Read the model definition and answer for the solid it produces. Units are mm, in the model's axes. A direction names the side the tool comes from. Give positions to 0.01 mm unless a question says otherwise; leave off trailing zeros. Order: outer loops, then holes, each group sorted by start corner. A loop starts at its lowest first (then second) coordinate and runs counter-clockwise, first axis right, second up.
Autodesk Inventor part; units mm, degrees
ref_plane "YZ Plane" through (0, 0, 0) normal (1, 0, 0) x (0, 1, 0)
ref_plane "XZ Plane" through (0, 0, 0) normal (0, 1, 0) x (-1, 0, 0)
ref_plane "XY Plane" through (0, 0, 0) normal (0, 0, 1) x (1, 0, 0)
sketch "Sketch1" plane through (0, 0, 0) normal (0, 1, 0) x (-1, 0, 0)
  line L0 (28, 44) -> (-28, 44)
  line L1 (-30, 42) -> (-30, -42)
  line L2 (-28, -44) -> (28, -44)
  line L3 (30, -42) -> (30, 42)
  line L4 (30, 44) -> (-30, -44) construction
  line L5 (-30, 44) -> (30, -44) construction
  line L6 (25, 42.5) -> (-25, 42.5)
  line L7 (-28, 39.5) -> (-28, -39.5)
  line L8 (-25, -42.5) -> (25, -42.5)
  line L9 (28, -39.5) -> (28, 39.5)
  line L10 (28, 42.5) -> (-28, -42.5) construction
  line L11 (-28, 42.5) -> (28, -42.5) construction
  arc A0 (25, -42.5) -> (28, -39.5) centre (25, -39.5) ccw
  arc A1 (-28, -39.5) -> (-25, -42.5) centre (-25, -39.5) ccw
  arc A2 (-25, 42.5) -> (-28, 39.5) centre (-25, 39.5) ccw
  arc A3 (28, 39.5) -> (25, 42.5) centre (25, 39.5) ccw
  arc A4 (-30, -42) -> (-28, -44) centre (-28, -42) ccw
  arc A5 (-28, 44) -> (-30, 42) centre (-28, 42) ccw
  arc A6 (28, -44) -> (30, -42) centre (28, -42) ccw
  arc A7 (30, 42) -> (28, 44) centre (28, 42) ccw
  point P0 (0, 0)
  dimension "d2" = 60
  dimension "d3" = 88
  dimension "d4" = 56
  dimension "d5" = 85
  dimension "d6" = 3
  dimension "d7" = 2
extrude "Extrusion1" add sketch "Sketch1" along normal blind 4 contours A7 L3 A6 L2 A4 L1 A5 L0 | A3 L9 A0 L8 A1 L7 A2 L6
extrude "Extrusion2" add sketch "Sketch1" against normal blind 8
sketch "Sketch2" plane through (28, 4, -44) normal (0, 0, -1) x (-1, 0, 0)
  line L0 (53, -12) -> (3, -12)
  line L1 (2, -1) -> (54, -1)
  line L2 (54, -1) -> (54, -12)
  line L3 (54, -12) -> (2, -12)
  line L4 (2, -12) -> (2, -1)
  line L5 (-2, -12) -> (-2, 0)
  line L6 (58, 0) -> (58, -12)
  point P0 (28, -4)
  dimension "d12" = 4
  dimension "d13" = 4
  dimension "d14" = 11
extrude "Extrusion3" cut sketch "Sketch2" against normal blind 19
sketch "Sketch3" plane through (28, 4, -44) normal (0, 0, -1) x (-1, 0, 0)
  line L0 (2, -1) -> (54, -1)
  line L1 (54, -1) -> (38, -1)
  line L2 (38, -1) -> (38, -3.5)
  line L3 (38, -3.5) -> (54, -3.5)
  line L4 (54, -3.5) -> (54, -1)
  line L5 (0, 0) -> (56, 0)
  line L6 (2, -1) -> (54, -1)
  line L7 (54, -1) -> (54, 0)
  line L8 (54, 0) -> (2, 0)
  line L9 (2, 0) -> (2, -1)
  point P0 (28, -4)
  point P1 (38, -1)
  dimension "d17" = 16
  dimension "d18" = 2.5
extrude "Extrusion4" add sketch "Sketch3" against normal blind 21 contours L0 L4 L3 L2
extrude "Extrusion5" cut sketch "Sketch3" against normal blind 5
sketch "Sketch4" plane through (30, 4, 42) normal (1, 0, 0) x (0, 0, -1)
  line L0 (86, -12) -> (86, 0)
  line L1 (84, -12) -> (0, -12)
  circle A0 centre (53.5, -14.5) radius 3.5
  point P0 (42, -4)
  point P1 (51.0505, -12)
  point P2 (55.9495, -12)
  dimension "d27" = 2.5
  dimension "d28" = 32.5
  dimension "d29" = 7
extrude "Extrusion6" cut sketch "Sketch4" against normal blind 10 contours L1 A0 picked at (52.8865, -11.841)
sketch "Sketch5" plane through (30, 4, 42) normal (1, 0, 0) x (0, 0, -1)
  line L0 (-4.9094, -13.7) -> (89.7531, -13.7)
  line L1 (84, -12) -> (55.9495, -12)
  point P0 (42, -4)
  dimension "d32" = 1.7
sketch "Sketch6" plane through (30, 4, 42) normal (1, 0, 0) x (0, 0, -1)
  line L0 (43, -10.0638) -> (43, -13.7)
  arc A0 (55.9495, -12) -> (51.0505, -12) centre (53.5, -14.5) ccw
  line L1 (35, -10.0638) -> (35, -13.7)
  line L2 (30, -13.7) -> (30, -10.0638)
  line L3 (22, -10.0638) -> (22, -13.7)
  line L4 (17, -10.0638) -> (17, -13.7)
  line L5 (7, -10.0638) -> (7, -13.7)
  line L6 (6.4702, -10.0638) -> (43, -10.0638)
  line L7 (-3.7275, -13.7) -> (104.8817, -13.7)
  line L8 (84, -12) -> (55.9495, -12)
  point P0 (42, -4)
  dimension "d33" = 10.5
  dimension "d34" = 8
  dimension "d35" = 5
  dimension "d36" = 8
  dimension "d37" = 5
  dimension "d38" = 10
  dimension "d39" = 1.7
extrude "Extrusion7" add sketch "Sketch6" against normal blind 2 contours L0 L7 L1 L6 | L2 L7 L3 L6 | L4 L7 L5 L6
fillet "Fillet1" radius 1 10 edges at (29.4142, 4, -43.4142) (27, 4, -44) (29.4142, 4, 43.4142) (0, 4, 44) (-29.4142, 4, 43.4142) (-30, 4, 0) (-29.4142, 4, -43.4142) (-27, 4, -44) (30, 4, 0) (0, 4, -39)
properties part number "Pi 4 Case  - Upper Panel"
1) The part is cut by section B-B on z = 38.5. Determine the outline of the cut face in (x, y).
Final values:
outline: (-30, -8) - (-28, -8) - (-28, 0) - (28, 0) - (28, -8) - (30, -8) - (30, 3) arc R1 ccw to (29, 4) - (-29, 4) arc R1 ccw to (-30, 3) - close
2) The part is cut by section A-A on x = -23.5. Determine the outline of the cut face in (y, z).
Final values:
outline: (-8, 42.5) - (0, 42.5) - (0, -25) - (0.5, -25) - (0.5, -39) - (3, -39) arc R1 ccw to (4, -38) - (4, 43) arc R1 ccw to (3, 44) - (-8, 44) - close
3) A tool of negligible diameter and unlimited length cuts with its end or side. For faces 1 (the face through (27, -2, -44)), 2 (the face through (-28, -4, -1)), 3 (the face through (29, -8, -5)), 4 (the face through (29, -9, 35)), 5 (the face through (29, -9, 7)), from which of +Z, -Z, +X, -X, +Y, -Y can it reach the whole face along a straight path? Write none if from no direction.
Final values:
face 1: -Z, +X, -X, +Y, -Y
face 2: -Y
face 3: -Z, +X, -X, -Y
face 4: +Z, +X, -X, -Y
face 5: +X, -X, -Y
4) The part is cut by section D-D on z = -34.5. Determine the outline of the cut face in (x, y).
Final values:
outline: (-30, -8) - (-28, -8) - (-28, 0) - (-26, 0) - (-26, 0.5) - (-10, 0.5) - (-10, 3) - (26, 3) - (26, 0) - (28, 0) - (28, -8) - (30, -8) - (30, 3) arc R1 ccw to (29, 4) - (-29, 4) arc R1 ccw to (-30, 3) - close
5) For a pull along X with two mould halves and no side action, classify faces 6 (the face through (29, -9, 12)), 7 (the face through (28, -4, 1)), 8 (the face through (0, -4, 42.5)), 9 (the face through (29.4, -2.42, 43.43)) as released by +X, released by -X, zero draft, split by the parting line, or undercut.
Final values:
face 6: zero draft
face 7: undercut
face 8: undercut
face 9: released by +X
6) Consider L1, parallel to X at y = -3, z = 21.5; L2, parallel to Z at x = -15, y = -1.5; L3, parallel to Y at x = -5, z = -4. Determine where each line is inside the solid, lowest interval first.
Final values:
L1: x = -30 to -28, 28 to 30
L2: z = 42.5 to 44
L3: y = 0 to 4
7) Given pin 1 (2 mm diameter, centred on x = 2.5, z = 5, fed in from -Y); pin 2 (0.8 mm diameter, centred on x = 29.5, y = -8.5, fed in from -Z); pin 3 (6 mm diameter, centred on x = 21.5, y = -2, fed in from -Z), each flat-ended and moving along its own axis, determine where each tip first touches the part or whether it passes through.
Final values:
pin 1: stops at y = 0
pin 2: stops at z = -1
pin 3: stops at z = -25
8) The part is cut by section C-C on y = -3.5. Determine the outline of the cut face in (x, z), and give its area (3 significant figures).
Final values:
outline: (-30, -42) arc R2 ccw to (-28, -44) - (-26, -44) - (-26, -42.33) arc R3 cw to (-28, -39.5) - (-28, 39.5) arc R3 cw to (-25, 42.5) - (25, 42.5) arc R3 cw to (28, 39.5) - (28, -39.5) arc R3 cw to (26, -42.33) - (26, -44) - (28, -44) arc R2 ccw to (30, -42) - (30, 42) arc R2 ccw to (28, 44) - (-28, 44) arc R2 ccw to (-30, 42) - close
area: 446 mm2
